from build123d import *

# Parameters (mm, degrees)
SKETCH019_R     = 1.5
PAD009_DEPTH    = 2
SKETCH020_W     = 55.95
SKETCH020_H     = 4
PAD010_DEPTH    = 1
CHAMFER002_SIZE = 1


with BuildPart() as obj1:
    # Sketch019 → Pad009 (new body)
    with BuildSketch(Plane(origin=(0, 0, 0), x_dir=(-1, 0, 0), z_dir=(0, 0, -1))):
        with BuildLine():
            Line((-31, 45.1), (58.15, 45.1))
            ThreePointArc((64.15, 39.1), (62.392641, 43.342641), (58.15, 45.1))
            Line((64.15, 39.1), (64.15, -1.000024))
            ThreePointArc((58.15, -7), (62.392639, -5.242656), (64.15, -1.000024))
            Line((58.15, -7), (-31, -7))
            ThreePointArc((-37, -1), (-35.242641, -5.242641), (-31, -7))
            Line((-37, -1), (-37, 39.1))
            ThreePointArc((-31, 45.1), (-35.242641, 43.342641), (-37, 39.1))
        make_face()
        with Locations((-32.414214, 40.514214)):
            Circle(SKETCH019_R, mode=Mode.SUBTRACT)
        with Locations((59.564214, 40.514214)):
            Circle(SKETCH019_R, mode=Mode.SUBTRACT)
        with Locations((59.564214, -2.414214)):
            Circle(SKETCH019_R, mode=Mode.SUBTRACT)
        with Locations((-32.414214, -2.414214)):
            Circle(SKETCH019_R, mode=Mode.SUBTRACT)
    extrude(amount=PAD009_DEPTH)

    # Sketch020 (on Face14 of Pad009) → Pad010 (join)
    with BuildSketch(Plane(origin=(0, 0, -2), x_dir=(1, 0, 0), z_dir=(0, 0, -1))):
        with Locations((-28.675, -2.5)):
            Rectangle(SKETCH020_W, SKETCH020_H)
        with Locations((-28.675, -35.6)):
            Rectangle(SKETCH020_W, SKETCH020_H)
        Polygon((5.5, -33.6), (5.5, -37.6), (13, -37.6), (13, -45.1), (24, -45.1), (24, -37.6), (30.5, -37.6), (30.5, -33.6), (30.5, -4.5), (30.5, -3.5), (5.5, -3.5), (5.5, -4.5), align=None)
    extrude(amount=PAD010_DEPTH)

    # Chamfer002
    chamfer002_edges = [obj1.edges().sort_by_distance(p)[0] for p in [
        (-58.064214, -2.414214, 0),
        (-58.064214, 40.514214, 0),
        (33.914214, 40.514214, 0),
        (33.914214, -2.414214, 0),
    ]]
    chamfer(chamfer002_edges, length=CHAMFER002_SIZE)


with BuildPart() as part_mirroring:
    # Part__Mirroring: instance of obj1
    add(obj1.part.mirror(Plane(origin=(0, 0, 0), x_dir=(0, 1, 0), z_dir=(0, 0, 1))))


solid = part_mirroring.part
Verification items for the finished model (mm, model axes). Coordinates: 2 decimals unless noted, no trailing zeros. Write each loop counter-clockwise with the first axis right and the second up, starting at its lowest first coordinate (ties: lowest second). Pieces come first, ordered by that corner, then holes. Notation, with made-up numbers: M 3.5,-26.5 L 25.5,-26.5 A21 ccw 25.5,10.5 Z; hole C 0,-11.75 d1. An arc over 180 degrees is marked long. One line per question, with ' | ' between items.
1) Sectioned sample at B-B on x = -49.5. Record the cut outline in (y, z), then the cut area to 3 significant figures.
Solutions:
outline: M -7,0 L 45.1,0 L 45.1,2 L 37.6,2 L 37.6,3 L 33.6,3 L 33.6,2 L 4.5,2 L 4.5,3 L 0.5,3 L 0.5,2 L -7,2 Z | area: 112 mm^2
2) Sectioned sample at D-D on x = 3.5. Record the cut outline in (y, z), then the cut area to 3 significant figures.
Solutions:
outline: M -7,0 L 45.1,0 L 45.1,2 L -7,2 Z | area: 104 mm^2
3) Depth check by flat-ended pin: pin 1 Ø4 at (x, y) = (32.41, 40.51) entering from -Z; pin 2 Ø5 at (x, y) = (-59.56, 40.51) entering from +Z; pin 3 Ø0.5 at (y, z) = (43, 2.5) entering from -X; pin 4 Ø6 at (x, y) = (-9.5, 9.5) entering from -Z. Enter the tip coordinate at first touch or a pass-through.
Solutions:
pin 1: z = 0.49 | pin 2: z = 2 | pin 3: x = 13 | pin 4: z = 0
4) Sectioned sample at C-C on y = 2.5. Record the cut outline in (x, z).
Solutions:
outline: M -64.15,0 L 37,0 L 37,2 L -0.7,2 L -0.7,3 L -56.65,3 L -56.65,2 L -64.15,2 Z
5) Release check for a two-part mould opening along X. For faces 1 (the face through (-62.439, 43.296, 0.986)), 2 (the face through (-14, 19, 0)), 3 (the face through (-60.995, 40.965, 1.493)), 4 (the face through (37, 19, 1)) record: +X half, -X half, draft (parallel to the pull), parting line (faces both ways), or undercut.
Solutions:
face 1: -X half | face 2: draft | face 3: undercut | face 4: +X half
6) Sectioned sample at A-A on y = 21.5. Record the cut outline in (x, z), then the cut area to 3 significant figures.
Solutions:
outline: M -64.15,0 L 37,0 L 37,2 L 30.5,2 L 30.5,3 L 5.5,3 L 5.5,2 L -64.15,2 Z | area: 227 mm^2
7) Material ranges on L1, parallel to Y at x = -51, z = 2.8; L2, parallel to X at y = 2, z = 2.05; L3, parallel to Y at x = 32, z = 1.1, recorded low to high.
Solutions:
L1: 0.5 to 4.5, 33.6 to 37.6 | L2: -56.65 to -0.7 | L3: -6.92 to -3.86, -0.97 to 39.07, 41.96 to 45.02
